Geometry: final body of the model. Coordinates: model frame, mm. A direction names the side the tool comes from. Give positions to 0.01 mm unless a question says otherwise; leave off trailing zeros. Loops run counter-clockwise (first coordinate to the right, second up) from the corner with the lowest first, then second, coordinate; pieces in that order, holes last.
1. Material intervals for line 1 along Z through (x, y) = (-1, 8); line 2 along Z through (x, y) = (-1, -10.5); line 3 along X through (y, z) = (-3, 39), sorted ascending.
2. First-contact query: P1, Ø6, axis at y = 3.5, z = 55.5, coming from the -X side; P2, Ø4, axis at y = -5.5, z = 16.5, coming from the +X side. Flat tips, straight axial feed; report the tip coordinate or a pass-through.
3. Section D-D, the plane z = 9. Output: boundary loops of the cut face in (x, y).
4. Section C-C, the plane z = 60.5. Output: boundary loops of the cut face in (x, y).
5. Section A-A, the plane x = 0. Output: boundary loops of the cut face in (y, z), then the cut area to 3 significant figures.
6. Draft query along Z for faces 1 (the face through (-9.54, 3, 11.92)), 2 (the face through (8.2, 0, 6)), 3 (the face through (0, 0, 0)). Return one class per face: +Z half, -Z half, draft (parallel to the pull), parting line (faces both ways), or undercut.
7. Access query for faces 4 (the face through (-11.99, 0.53, 53.5)), 5 (the face through (5, 9, 18)), 6 (the face through (-7.81, -1.73, 4.99)). Directions: +Z, -Z, +X, -X, +Y, -Y. A direction counts if a zero-diameter tool reaches every point of the face in a straight line with its end or side. Return the directions, or none.
from build123d import *

# Parameters (mm, degrees)
SKETCH1_R           = 12
BOSS_EXTRUDE1_DEPTH = 90
SKETCH2_R           = 12
SKETCH2_R_2         = 10
CUT_EXTRUDE2_DEPTH  = 18
SKETCH3_W           = 2
SKETCH3_H           = 2


with BuildPart() as part:
    # Sketch1 → Boss-Extrude1 (new body)
    with BuildSketch(Plane.XY):
        Circle(SKETCH1_R)
    extrude(amount=BOSS_EXTRUDE1_DEPTH)

    # Sketch2 → Cut-Extrude2 (cut)
    with BuildSketch(Plane(origin=(0, 0, 0), x_dir=(-1, 0, 0), z_dir=(0, 0, -1))):
        Circle(SKETCH2_R)
        Circle(SKETCH2_R_2, mode=Mode.SUBTRACT)
    extrude(amount=-CUT_EXTRUDE2_DEPTH, mode=Mode.SUBTRACT)

    # Sketch3 → Cut-Revolve1 (revolve, cut)
    with BuildSketch(Plane(origin=(0, 0, 0), x_dir=(0, 0, -1), z_dir=(1, 0, 0))):
        with Locations((-5, 9)):
            Rectangle(SKETCH3_W, SKETCH3_H)
    revolve(axis=Axis((0, 0, 18), (0, 0, -1)), mode=Mode.SUBTRACT)


solid = part.part
Answers below:
1. line 1: z = 0 to 4, 6 to 90
1. line 2: z = 18 to 90
1. line 3: x = -11.62 to 11.62
2. P1: stops at x = -11.99
2. P2: stops at x = 11.25
3. outline: circle Ø20 at (0, 0)
4. outline: circle Ø24 at (0, 0)
5. outline: (-12, 18) - (-10, 18) - (-10, 6) - (-8, 6) - (-8, 4) - (-10, 4) - (-10, 0) - (10, 0) - (10, 4) - (8, 4) - (8, 6) - (10, 6) - (10, 18) - (12, 18) - (12, 90) - (-12, 90) - close
5. area: 2,080 mm2
6. face 1: draft
6. face 2: undercut
6. face 3: -Z half
7. face 4: +Z, -Z
7. face 5: -Z
7. face 6: none
